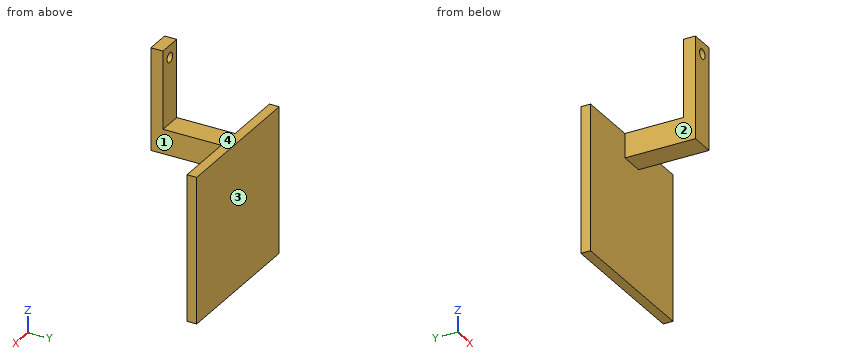
```python
from build123d import *

# Parameters (mm, degrees)
SKETCH1_W           = 30
SKETCH1_H           = 30
BOSS_EXTRUDE1_DEPTH = 2
BOSS_EXTRUDE2_DEPTH = 14.5
SKETCH3_W           = 5
SKETCH3_H           = 2.5
BOSS_EXTRUDE3_DEPTH = 16
SKETCH4_R           = 1
CUT_EXTRUDE1_DEPTH  = 5


with BuildPart() as part:
    # Sketch1 → Boss-Extrude1 (new body)
    with BuildSketch(Plane(origin=(0, 0, 0), x_dir=(1, 0, 0), z_dir=(0, 1, 0))):
        Rectangle(SKETCH1_W, SKETCH1_H)
    extrude(amount=BOSS_EXTRUDE1_DEPTH)

    # Sketch2 → Boss-Extrude2 (add)
    with BuildSketch(Plane.XZ):
        Polygon((2.5, 15), (0, 15), (-2.5, 15), (-2.5, 10), (2.5, 10), align=None)
    extrude(amount=BOSS_EXTRUDE2_DEPTH)

    # Sketch3 → Boss-Extrude3 (add)
    with BuildSketch(Plane.XY.offset(15)):
        with Locations((0, -13.25)):
            Rectangle(SKETCH3_W, SKETCH3_H)
    extrude(amount=BOSS_EXTRUDE3_DEPTH)

    # Sketch4 → Cut-Extrude1 (cut)
    with BuildSketch(Plane(origin=(0, -14.5, 0), x_dir=(-1, 0, 0), z_dir=(0, -1, 0))):
        with Locations((0, -28.5)):
            Circle(SKETCH4_R)
    extrude(amount=-CUT_EXTRUDE1_DEPTH, mode=Mode.SUBTRACT)


solid = part.part
```
Part model, mm, in its own coordinate system. Face numbers are marked on the shaded views. A direction names the side the tool comes from. Round coordinates to 2 decimals unless told otherwise and drop trailing zeros. Write each loop counter-clockwise with the first axis right and the second up, starting at its lowest first coordinate (ties: lowest second). Pieces come first, ordered by that corner, then holes. Notation, with made-up numbers: (32.5, -1.5) -> (85.5, -1.5) arc R18 cw to (85.5, 23.5) -> close; hole circle Ø9 at (8, 86.25). An arc over 180 degrees is marked (long way). Return JSON: item names as keys, results as strings. Group by question number.
Q1. Which spindle directions (+Z, -Z, +X, -X, +Y, -Y) get a long thin tool onto all of the face, cutting with end or side? Do the marked faces 1, 2, 3 and 4. Say none if no direction does.
Q2. Saw through at B-B on x = 0. Write the cut outline in (y, z).
Q3. Saw through at C-C on y = -13. Write the cut outline in (x, z).
Q4. Saw through at D-D on x = -11.5. Write the cut outline in (y, z), plus the area to 3 significant figures.
Q5. Pin check, flat tips, straight feed: pin 1 (8 mm diameter, centred on x = 8.5, z = 25, fed in from -Y); pin 2 (7 mm diameter, centred on x = 4.5, y = -4.5, fed in from +Z); pin 3 (2.5 mm diameter, centred on x = 1, z = 19.5, fed in from +Y); pin 4 (5.5 mm diameter, centred on x = 0.5, y = -9.5, fed in from -Z). Stop position of each tip, or through.
Q6. Saw through at A-A on z = 28.5. Write the cut outline in (x, y), plus the area to 3 significant figures.
Q7. Probe L1, parallel to Z at x = 0, y = -13; L2, parallel to X at y = -13.25, z = 28.5; L3, parallel to Y at x = 4, z = -5.5. List the from-to ranges inside material, lowest first. Write a range as [from, to].
Answer:
{
 "1": {"face 1": "+Z, -Z, +X, -Y", "face 2": "+Z, -Z, -X, -Y", "face 3": "+Z, -Z, +X, -X, +Y", "face 4": "+Z, +X, -X, +Y"},
 "2": {"outline": "(-14.5, 10) -> (0, 10) -> (0, -15) -> (2, -15) -> (2, 15) -> (-12, 15) -> (-12, 27.5) -> (-14.5, 27.5) -> close; (-14.5, 29.5) -> (-12, 29.5) -> (-12, 31) -> (-14.5, 31) -> close"},
 "3": {"outline": "(-2.5, 10) -> (2.5, 10) -> (2.5, 31) -> (-2.5, 31) -> close; hole circle Ø2 at (0, 28.5)"},
 "4": {"outline": "(0, -15) -> (2, -15) -> (2, 15) -> (0, 15) -> close", "area": "60.0 mm2"},
 "5": {"pin 1": "through", "pin 2": "z = 15", "pin 3": "y = -12", "pin 4": "z = 10"},
 "6": {"outline": "(-2.5, -14.5) -> (-1, -14.5) -> (-1, -12) -> (-2.5, -12) -> close; (1, -14.5) -> (2.5, -14.5) -> (2.5, -12) -> (1, -12) -> close", "area": "7.50 mm2"},
 "7": {"L1": "[10, 27.5], [29.5, 31]", "L2": "[-2.5, -1], [1, 2.5]", "L3": "[0, 2]"}
}
